The listing builds one solid part. Answer for the finished solid, in the listing's coordinates (mm). A direction names the side the tool comes from. Coordinates: 2 decimals unless noted, no trailing zeros. Write each loop counter-clockwise with the first axis right and the second up, starting at its lowest first coordinate (ties: lowest second). Pieces come first, ordered by that corner, then holes. Notation, with made-up numbers: M -34.5,62 L 24.5,62 A25 ccw 24.5,81 Z; hole C 22.25,-24 d6. An arc over 180 degrees is marked long. Answer as CSV lines item,"result".
```python
from build123d import *

# Parameters (mm, degrees)
SKETCH_R        = 5
PAD_DEPTH       = 2
SKETCH001_R     = 4
PAD001_DEPTH    = 3
POCKET_DEPTH    = 3
SKETCH003_R     = 0.5
POCKET001_DEPTH = 5.001
FILLET_R        = 0.5
FILLET001_R     = 0.5
FILLET002_R     = 0.5
FILLET003_R     = 0.2


with BuildPart() as part:
    # Sketch → Pad (new body)
    with BuildSketch(Plane.XY):
        Circle(SKETCH_R)
    extrude(amount=PAD_DEPTH)

    # Sketch001 (on Face3 of Pad) → Pad001 (join)
    with BuildSketch(Plane.XY.offset(2)):
        Circle(SKETCH001_R)
    extrude(amount=PAD001_DEPTH)

    # Sketch002 (on Face5 of Pad001) → Pocket (cut)
    with BuildSketch(Plane.XY.offset(5)):
        with BuildLine():
            ThreePointArc((-1, 2.2), (-3.2, 0), (-1, -2.2))
            Line((-1, -2.2), (1, -2.2))
            ThreePointArc((1, -2.2), (3.2, 0), (1, 2.2))
            Line((-1, 2.2), (1, 2.2))
        make_face()
    extrude(amount=-POCKET_DEPTH, mode=Mode.SUBTRACT)

    # Sketch003 (on Face5 of Pocket) → Pocket001 (cut, through all)
    with BuildSketch(Plane.XY.offset(5)):
        with Locations((-1.5, 0)):
            Circle(SKETCH003_R)
        with Locations((1.5, 0)):
            Circle(SKETCH003_R)
    extrude(amount=-POCKET001_DEPTH, mode=Mode.SUBTRACT)

    # Fillet
    fillet_edges = [part.edges().sort_by_distance(p)[0] for p in [
        (-4, 0, 2),
    ]]
    fillet(fillet_edges, radius=FILLET_R)

    # Fillet001
    fillet001_edges = [part.edges().sort_by_distance(p)[0] for p in [
        (-2, 0, 2),
    ]]
    fillet(fillet001_edges, radius=FILLET001_R)

    # Fillet002
    fillet002_edges = [part.edges().sort_by_distance(p)[0] for p in [
        (1, 0, 2),
    ]]
    fillet(fillet002_edges, radius=FILLET002_R)

    # Fillet003
    fillet003_edges = [part.edges().sort_by_distance(p)[0] for p in [
        (-4, 0, 5),
        (-3.2, 0, 5),
        (0, -2.2, 5),
        (3.2, 0, 5),
        (0, 2.2, 5),
    ]]
    fillet(fillet003_edges, radius=FILLET003_R)


solid = part.part
```
Q1. The mould has two halves that part along X. Classify faces 3 (the flat face through (-1, 3, 5)), 4 (the flat face through (0, 0, 2)), 5 (the cylindrical face through (-0.867, -3.905, 3.634)): pulls with the +X half, pulls with the -X half, needs draft (parallel to the pull), parting line crosses it, or undercut.
Output:
face 3,"needs draft"
face 4,"undercut"
face 5,"parting line crosses it"
Q2. For faces 1 (the cylindrical face through (-3.2, 0, 3.4)), 2 (the cylindrical face through (-1.08, -4.88, 0.99)), determine the directions among +Z, -Z, +X, -X, +Y, -Y from which every point of the face is accessible in a straight line to the end or side of a thin tool.
Output:
face 1,"+Z"
face 2,"+Z, -Z"
Q3. Find section A-A (y = 0). Count the separate pieces of the cut face and the enclosed holes in it, and give its area (3 significant figures).
Output:
separate pieces,"3"
enclosed holes,"0"
area,"20.7 mm2"
Q4. Find section C-C (z = 0.7). Give the vertices of the cut face in (x, y), and give its area (3 significant figures).
Output:
outline,"C 0,0 d10; hole C -1.5,0 d1; hole C 1.5,0 d1"
area,"77.0 mm2"
Q5. Find section B-B (z = 3.7). Give the vertices of the cut face in (x, y).
Output:
outline,"C 0,0 d8; hole M -1,-2.2 L 1,-2.2 A2.2 ccw 1,2.2 L -1,2.2 A2.2 ccw Z"
Q6. Straight lines are drawn through the part: line 1 (Z direction, x = 3.25, y = -2.5); line 2 (Z direction, x = -2.25, y = 1.5); line 3 (Y direction, x = -1.5, z = 0.7). For each, find the intervals that lie inside material, in ascending order.
Output:
line 1,"0 to 2.2"
line 2,"0 to 2"
line 3,"-4.77 to -0.5, 0.5 to 4.77"
Q7. Flat-ended cylindrical pins translate along their axes: pin 1 Ø4 at (x, y) = (3, -2.5) entering from +Z; pin 2 Ø1 at (x, z) = (0.5, 3.5) entering from +Y; pin 3 Ø1.5 at (x, z) = (-1, 2.5) entering from +Y. Find the tip coordinate at first contact, or state that the pin passes through.
Output:
pin 1,"z = 5"
pin 2,"y = 4"
pin 3,"y = 4.98"
Q8. Find section D-D (z = 1.8). Give the vertices of the cut face in (x, y).
Output:
outline,"C 0,0 d10; hole C -1.5,0 d1.2; hole C 1.5,0 d1.2"
